Geometry check sheet. Reference: the model listing, model coordinates, mm. Round coordinates to 2 decimals unless told otherwise and drop trailing zeros. Loops run counter-clockwise (first coordinate to the right, second up) from the corner with the lowest first, then second, coordinate; pieces in that order, holes last. Notation, with made-up numbers: (13.5, -11) - (70.5, -11) arc R16 cw to (70.5, 6) - close; hole circle Ø8 at (-10.75, 83.5). An arc over 180 degrees is marked (long way). Write item = value, one per line.
```python
from build123d import *

# Parameters (mm, degrees)
SKETCH1_W           = 20
SKETCH1_H           = 75
BOSS_EXTRUDE1_DEPTH = 3
CUT_EXTRUDE1_START  = -4
SKETCH2_W           = 5
SKETCH2_H           = 3
CUT_EXTRUDE1_DEPTH  = 5


with BuildPart() as part:
    # Sketch1 → Boss-Extrude1 (new body)
    with BuildSketch(Plane(origin=(0, 0, 0), x_dir=(1, 0, 0), z_dir=(0, 1, 0))):
        Rectangle(SKETCH1_W, SKETCH1_H)
    extrude(amount=BOSS_EXTRUDE1_DEPTH)

    # Sketch2 → Cut-Extrude1 (cut)
    with BuildSketch(Plane.XZ.offset(CUT_EXTRUDE1_START)):
        with Locations((-5, 36)):
            Rectangle(SKETCH2_W, SKETCH2_H)
    cut_extrude1 = extrude(amount=CUT_EXTRUDE1_DEPTH, mode=Mode.SUBTRACT)

    # Mirror1: Cut-Extrude1 across plane
    add(cut_extrude1.mirror(Plane(origin=(0, 0, 0), x_dir=(0, 0, 1), z_dir=(1, 0, 0))), mode=Mode.SUBTRACT)


solid = part.part
```
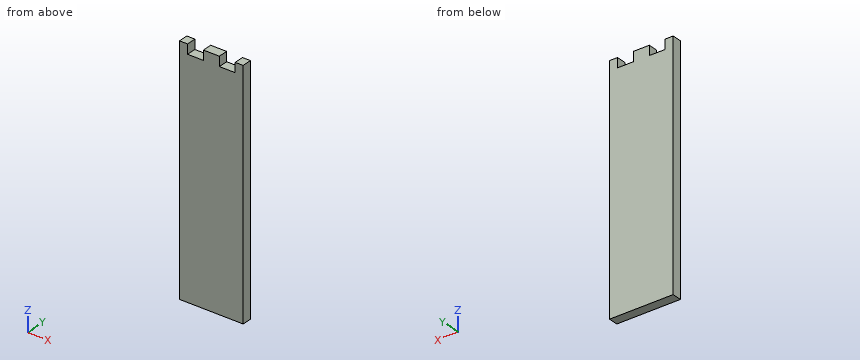
(1) Section check A-A (y = 1.7). Enter the section's corners in (x, z).
Answers follow:
outline = (-10, -37.5) - (10, -37.5) - (10, 37.5) - (7.5, 37.5) - (7.5, 34.5) - (2.5, 34.5) - (2.5, 37.5) - (-2.5, 37.5) - (-2.5, 34.5) - (-7.5, 34.5) - (-7.5, 37.5) - (-10, 37.5) - close
(2) Gauge pin test, flat ends, axial feed: pin 1 (1.5 mm diameter, centred on x = -4, y = 2, fed in from +Z); pin 2 (10 mm diameter, centred on x = 4.5, z = 8.5, fed in from -Y). Record the tip position at first contact, or that the pin passes through.
Answers follow:
pin_1 = 34.5
pin_2 = 0
(3) Scan line: L1, parallel to Z at x = 4.5, y = 1.45. Record every from-to range of solid material in increasing order. Write a range as [from, to].
Answers follow:
L1 = [-37.5, 34.5]
(4) Section check B-B (x = 4.75). Enter the section's corners in (y, z), then the cut area to 3 significant figures.
Answers follow:
outline = (0, -37.5) - (3, -37.5) - (3, 34.5) - (0, 34.5) - close
area = 216 mm²
